Part model, mm, in its own coordinate system. Face numbers are marked on the shaded views. Give positions to 0.01 mm unless a question says otherwise; leave off trailing zeros. Write each loop counter-clockwise with the first axis right and the second up, starting at its lowest first coordinate (ties: lowest second). Pieces come first, ordered by that corner, then holes. Notation, with made-up numbers: (-15, 28) - (27, 28) arc R30 ccw to (27, 56) - close; hole circle Ø5 at (69, 85). An arc over 180 degrees is marked (long way). Answer in a Markdown table with one row per item. Add a question column.
1. Pull direction Y, two halves, no side cores. Call the marked faces 1, 2 and 3: released by +Y, released by -Y, zero draft, split by the parting line, or undercut.
2. Drop a flat-ended pin along its axis: pin 1 Ø4.5 at (x, y) = (-15.5, 15.5) entering from +Z. Give the stop position or say it passes through.
3. Band-saw the part on D-D on z = 3. Write the cut outline in (x, y), plus the area to 3 significant figures.
4. Probe line 1 along X through (y, z) = (17, 1.25); line 2 along Y through (x, z) = (0, 2); line 3 along X through (y, z) = (-16.5, 4). List the from-to ranges inside material, lowest first.
5. Band-saw the part on B-B on x = -15.5. Write the cut outline in (y, z), plus the area to 4 significant figures.
6. Band-saw the part on A-A on y = 0. Write the cut outline in (x, z).
```python
from build123d import *

# Parameters (mm, degrees)
SKETCH1_W                = 42.3
SKETCH1_H                = 42.3
SKETCH1_R                = 12.5
BOSS_EXTRUDE1_DEPTH      = 7
CHAMFER1_SIZE            = 3
M3_CLEARANCE_HOLE1_D     = 3.4
M3_CLEARANCE_HOLE1_DEPTH = 7.5
M3_CLEARANCE_HOLE1_TIP   = 1.021463052


with BuildPart() as part:
    # Sketch1 → Boss-Extrude1 (new body)
    with BuildSketch(Plane.XY):
        Rectangle(SKETCH1_W, SKETCH1_H)
        Circle(SKETCH1_R, mode=Mode.SUBTRACT)
    extrude(amount=BOSS_EXTRUDE1_DEPTH)

    # Chamfer1
    chamfer1_edges = [part.edges().sort_by_distance(p)[0] for p in [
        (21.15, -21.15, 3.5),
        (-21.15, -21.15, 3.5),
        (-21.15, 21.15, 3.5),
        (21.15, 21.15, 3.5),
    ]]
    chamfer(chamfer1_edges, length=CHAMFER1_SIZE)

    # M3 Clearance Hole1
    with Locations(Plane.XY.offset(7)):
        with Locations((15.5, 15.5), (-15.5, 15.5), (-15.5, -15.5), (15.5, -15.5)):
            Hole(M3_CLEARANCE_HOLE1_D / 2, depth=M3_CLEARANCE_HOLE1_DEPTH)
            with Locations((0, 0, -(M3_CLEARANCE_HOLE1_DEPTH + M3_CLEARANCE_HOLE1_TIP / 2))):  # 118° drill point
                Cone(0, M3_CLEARANCE_HOLE1_D / 2, M3_CLEARANCE_HOLE1_TIP, mode=Mode.SUBTRACT)


solid = part.part
```
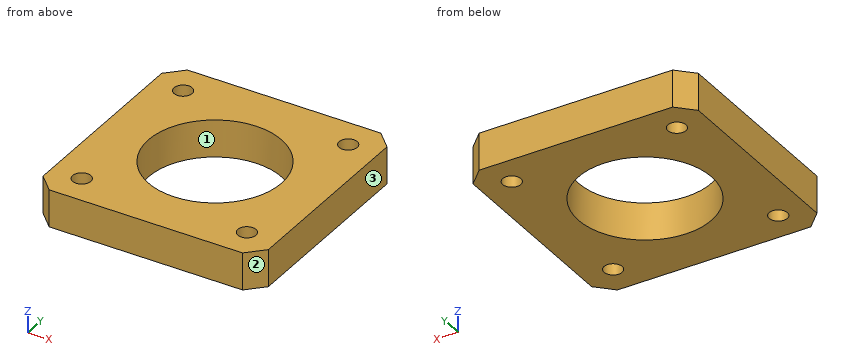
Values:
| question | item | result |
|---|---|---|
| 1 | face 1 | undercut |
| 1 | face 2 | released by -Y |
| 1 | face 3 | zero draft |
| 2 | pin 1 | stops at z = 7 |
| 3 | outline | (-21.15, -18.15) - (-18.15, -21.15) - (18.15, -21.15) - (21.15, -18.15) - (21.15, 18.15) - (18.15, 21.15) - (-18.15, 21.15) - (-21.15, 18.15) - close; hole circle Ø3.4 at (-15.5, -15.5); hole circle Ø3.4 at (-15.5, 15.5); hole circle Ø25 at (0, 0); hole circle Ø3.4 at (15.5, -15.5); hole circle Ø3.4 at (15.5, 15.5) |
| 3 | area | 1,240 mm² |
| 4 | line 1 | x = -21.15 to -16.3, -14.7 to 14.7, 16.3 to 21.15 |
| 4 | line 2 | y = -21.15 to -12.5, 12.5 to 21.15 |
| 4 | line 3 | x = -21.15 to -16.87, -14.13 to 14.13, 16.87 to 21.15 |
| 5 | outline | (-21.15, 0) - (-17.2, 0) - (-17.2, 7) - (-21.15, 7) - close; (-13.8, 0) - (13.8, 0) - (13.8, 7) - (-13.8, 7) - close; (17.2, 0) - (21.15, 0) - (21.15, 7) - (17.2, 7) - close |
| 5 | area | 248.5 mm² |
| 6 | outline | (-21.15, 0) - (-12.5, 0) - (-12.5, 7) - (-21.15, 7) - close; (12.5, 0) - (21.15, 0) - (21.15, 7) - (12.5, 7) - close |
